```python
from build123d import *

# Parameters (mm, degrees)
SKETCH1_W           = 10.8966
SKETCH1_H           = 12.065
BOSS_EXTRUDE1_DEPTH = 9.652
SKETCH2_R           = 1.0795
BOSS_EXTRUDE2_DEPTH = 3.048
SKETCH6_R           = 1.524
SKETCH7_R           = 1.0795
SKETCH8_W           = 14.3764
SKETCH8_H           = 21.5392
BOSS_EXTRUDE3_DEPTH = 1.5748


with BuildPart() as part:
    # Sketch1 → Boss-Extrude1 (new body)
    with BuildSketch(Plane(origin=(0, 0, 0), x_dir=(1, 0, 0), z_dir=(0, 1, 0))):
        with Locations((5.4483, 6.0325)):
            Rectangle(SKETCH1_W, SKETCH1_H)
    extrude(amount=BOSS_EXTRUDE1_DEPTH)

    # Sketch2 → Boss-Extrude2 (add)
    with BuildSketch(Plane.ZY):
        with Locations(Location((-8.1915, 7.6835, 0), (0, 0, 180))):
            Circle(SKETCH2_R)
        with Locations(Location((-3.8735, 1.9685, 0), (0, 0, 180))):
            Circle(SKETCH2_R)
    extrude(amount=BOSS_EXTRUDE2_DEPTH)

    # Loft1: read off the stored shape, not the designer's step
    # Loft1: loft between two sections, ruled curve by curve
    loft1_from = [
        Edge.make_bspline([(-3.048, 9.153232542, -7.788433932), (-3.048, 9.959364678, -10.727899016), (-3.048, 7.019899594, -11.534031152), (-3.048, 6.213767458, -8.594566068), (-3.048, 5.407635322, -5.655100984), (-3.048, 8.347100406, -4.848968848), (-3.048, 9.153232542, -7.788433932)], [0, 0, 0, 0, 0.5, 0.5, 0.5, 1, 1, 1, 1], 3, [1, 0.333333333, 0.333333333, 1, 0.333333333, 0.333333333, 1]),
    ]
    loft1_to = [
        Edge.make_bspline([(-6.223, 8.482388093, -7.465484805), (-6.223, 9.934418484, -9.063260992), (-6.223, 8.336642297, -10.515291382), (-6.223, 6.884611907, -8.917515195), (-6.223, 5.432581516, -7.319739008), (-6.223, 7.030357703, -5.867708618), (-6.223, 8.482388093, -7.465484805)], [0, 0, 0, 0, 0.5, 0.5, 0.5, 1, 1, 1, 1], 3, [1, 0.333333333, 0.333333333, 1, 0.333333333, 0.333333333, 1]),
    ]
    loft1 = Solid(Shell([*[Face.make_surface_from_curves(loft1_from[k], loft1_to[k]) for k in range(1)], Face(Wire(loft1_from)), Face(Wire(loft1_to))]))
    add(loft1)

    # Sketch6 → Loft2 section 0
    with BuildSketch(Plane.ZY.offset(3.048)):
        with Locations((-3.8735, 1.9685)):
            Circle(SKETCH6_R)
    # Sketch7 → Loft2 section 1
    with BuildSketch(Plane.ZY.offset(6.223)):
        with Locations((-3.8735, 1.9685)):
            Circle(SKETCH7_R)
    loft()

    # Sketch8 → Boss-Extrude3 (add)
    with BuildSketch(Plane.XZ):
        with Locations((5.4483, -6.0325)):
            Rectangle(SKETCH8_W, SKETCH8_H)
    extrude(amount=BOSS_EXTRUDE3_DEPTH)


solid = part.part
```
Geometry: final body of the model. Coordinates: model frame, mm. A direction names the side the tool comes from. Give positions to 0.01 mm unless a question says otherwise; leave off trailing zeros. Write each loop counter-clockwise with the first axis right and the second up, starting at its lowest first coordinate (ties: lowest second). Pieces come first, ordered by that corner, then holes.
1. Draft query along X for faces 1 (the flat face through (5, -1, 4.737)), 2 (the flat face through (12.636, -1, -6)), 3 (the flat face through (-3.048, 1, -3)), 4 (the conical face through (-5.01, 2.34, -2.68)). Return one class per face: released by +X, released by -X, zero draft, split by the parting line, or undercut.
2. Section query C-C, the plane x = 8.75. Return loops of the section in (y, z) (3 decimals).
3. Section query B-B, the plane x = -0.5. Return loops of the section in (y, z).
4. Line query: probe 1 along Y at (x, z) = (5, -12.5); probe 2 along Z at (x, y) = (6.25, 1) (3 decimals); probe 3 along X at (y, z) = (9, -1.5). Output: solid intervals per line, ascending.
5. Pin query (flat end, axial travel): P1, Ø1.5, axis at y = 2.5, z = -4.5, coming from the +X side; P2, Ø1.3, axis at y = -1, z = -9.5, coming from the -X side; P3, Ø1, axis at y = 4.5, z = -14, coming from the -X side; P4, Ø5, axis at x = 4, y = 4, coming from the +Z side. Return the tip coordinate at first contact, or that it passes through.
6. Section query A-A, the plane z = -0.75. Return loops of the section in (x, y), then the cut area to 3 significant figures.
7. Reachability of faces 5 (the flat face through (5, 5, 0)), 6 (the flat face through (5, 5, -12.065)), 7 (the cylindrical face through (-1.503, 8.737, -7.957)), 8 (the flat face through (10.897, 5, -6)) from +Z, -Z, +X, -X, +Y, -Y: full face, straight path, thin tool, end or side. Return the list, or none.
8. Section query D-D, the plane y = 4.75. Return loops of the section in (x, z) (3 decimals).
Computed:
1. face 1: zero draft
1. face 2: released by +X
1. face 3: undercut
1. face 4: released by -X
2. outline: (-1.575, -16.802) - (0, -16.802) - (0, -12.065) - (9.652, -12.065) - (9.652, 0) - (0, 0) - (0, 4.737) - (-1.575, 4.737) - close
3. outline: (-1.57, -16.8) - (0, -16.8) - (0, 4.74) - (-1.57, 4.74) - close; circle Ø2.16 at (1.97, -3.87); circle Ø2.16 at (7.68, -8.19)
4. probe 1: y = -1.57 to 0
4. probe 2: z = -12.065 to 0
4. probe 3: x = 0 to 10.9
5. P1: stops at x = 10.9
5. P2: stops at x = -1.74
5. P3: passes through
5. P4: stops at z = 0
6. outline: (-1.74, -1.57) - (12.64, -1.57) - (12.64, 0) - (10.9, 0) - (10.9, 9.65) - (0, 9.65) - (0, 0) - (-1.74, 0) - close
6. area: 128 mm2
7. face 5: +Z, +X, -X, +Y
7. face 6: -Z, +X, -X, +Y
7. face 7: none
7. face 8: +Z, -Z, +X, +Y
8. outline: (0, -12.065) - (10.897, -12.065) - (10.897, 0) - (0, 0) - close
